from build123d import *

# Parameters (mm, degrees)
SKETCH_1_R      = 1.25
EXTRUDE_1_DEPTH = 3
FILLET_2_R      = 2.5


with BuildPart() as part:
    # Эскиз1 → Бобышка-Вытянуть1 (new body)
    with BuildSketch(Plane.XY):
        with BuildLine():
            Line((-12, -2), (-4.85412196, -2))
            ThreePointArc((-4.85412196, -2), (0, 5.25), (4.85412196, -2))
            Line((4.85412196, -2), (8.261355821, -2))
            ThreePointArc((8.261355821, -2), (2, 8.261355821), (-8.261355821, 2))
            Line((-8.261355821, 2), (-12, 2))
            ThreePointArc((-12, 2), (-14, 0), (-12, -2))
        make_face()
        with Locations((-12, 0)):
            Circle(SKETCH_1_R, mode=Mode.SUBTRACT)
    extrude(amount=EXTRUDE_1_DEPTH)

    # Скругление2
    # the kernel refuses this fillet: 2.5 mm, written as the material it adds along each edge
    with BuildSketch(Plane(origin=(-8.261355821, 2, 0), x_dir=(0.3235599082125896, 0.9462076863973683, 0), z_dir=(0, 0, 1))) as fillet_2_piece_1:
        with BuildLine():
            CenterArc((1.790852834, 2.489434763), FILLET_2_R, 198.878350274, 65.852260083)
            Line((-0.574666382, 1.680534992), (0, 0))
            ThreePointArc((0, 0), (0.780628158, 0.035921806), (1.561256317, 0))
        make_face()
    extrude(amount=3)
    # the kernel refuses this fillet: 2.5 mm, written as the material it takes off along each edge
    with BuildSketch(Plane(origin=(8.261355821, -2, -6.790979044), x_dir=(-1, 0, 0), z_dir=(0, 0, 1))) as fillet_2_2_piece_1:
        with BuildLine():
            CenterArc((2.282225449, -2.5), FILLET_2_R, 90, 94.780191847)
            ThreePointArc((-0.209078872, -2.708333333), (-0.21342859, -1.345760603), (0, 0))
            Line((0, 0), (2.282225449, 0))
        make_face()
    extrude(amount=16.581958087, mode=Mode.SUBTRACT)
    with BuildSketch(Plane(origin=(4.85412196, -2, -7.199330473), x_dir=(0.16240998892159433, 0.9867233632069768, 0), z_dir=(0, 0, 1))) as fillet_2_2_piece_2:
        with BuildLine():
            CenterArc((2.934505681, -2.435474059), FILLET_2_R, 103.045879434, 86.300928937)
            Line((0.467697273, -2.841499031), (0, 0))
            ThreePointArc((0, 0), (1.185088833, -0.135504477), (2.370177665, 0))
        make_face()
    extrude(amount=17.398660947, mode=Mode.SUBTRACT)
    with BuildSketch(Plane(origin=(-4.85412196, -2, -7.199330473), x_dir=(-1, 0, 0), z_dir=(0, 0, 1))) as fillet_2_2_piece_3:
        with BuildLine():
            CenterArc((2.879732189, -2.5), FILLET_2_R, 90, 86.300928937)
            ThreePointArc((0.384940528, -2.338709677), (0.326175697, -1.147347558), (0, 0))
            Line((0, 0), (2.879732189, 0))
        make_face()
    extrude(amount=17.398660947, mode=Mode.SUBTRACT)


solid = part.part
Read the model definition and answer for the solid it produces. Units are mm, in the model's axes. A direction names the side the tool comes from. Give positions to 0.01 mm unless a question says otherwise; leave off trailing zeros. Write each loop counter-clockwise with the first axis right and the second up, starting at its lowest first coordinate (ties: lowest second). Pieces come first, ordered by that corner, then holes. Notation, with made-up numbers: (39.25, 80.25) - (56.25, 80.25) arc R14 ccw to (56.25, 97.25) - close; hole circle Ø11 at (37.25, 45.25). An arc over 180 degrees is marked (long way). Answer in a Markdown table with one row per item. Add a question column.
Item 1: Section D-D, the plane x = 0 is taken. Write down the section's boundary in (y, z), and give its area (3 significant figures).
Item 2: Determine the mould class of faces 4 (the face through (-13.25, 0.05, 1.48)), 5 (the face through (-6, -1.3, 1.5)), 6 (the face through (-3, 5, 3)) for opening direction Y: pulls with the +Y half, pulls with the -Y half, needs draft (parallel to the pull), parting line crosses it, or undercut.
Item 3: Section A-A, the plane z = 1.6 is taken. Write down the section's boundary in (x, y), and give its area (3 significant figures).
Item 4: Flat-ended cylindrical pins translate along their axes: P1, Ø1, axis at y = 5, z = 0.5, coming from the -X side; P2, Ø1, axis at x = -10.5, z = 1.5, coming from the +Y side; P3, Ø1, axis at x = -4.5, z = 1, coming from the +Y side. Find the tip coordinate at first contact, or state that the pin passes through.
Item 5: Find the intervals of material crossed by L1, parallel to X at y = 0.5, z = 1.6; L2, parallel to Y at x = -12, z = 0.95; L3, parallel to X at y = -1, z = 1.2, in increasing order.
Item 6: A tool of negligible diameter and unlimited length cuts with its end or side. For faces 1 (the face through (5.71, -0.97, 1.48)), 2 (the face through (-11, 2, 1)), 3 (the face through (-10, -2, 1)), from which of +Z, -Z, +X, -X, +Y, -Y can it reach the whole face along a straight path? Write none if from no direction.
Item 7: Section C-C, the plane y = 0 is taken. Write down the section's boundary in (x, z), and give its area (3 significant figures).
Item 8: Section B-B, the plane y = 3.25 is taken. Write down the section's boundary in (x, z).
Recorded:
| question | item | result |
|---|---|---|
| 1 | outline | (5.25, 0) - (8.5, 0) - (8.5, 3) - (5.25, 3) - close |
| 1 | area | 9.75 mm2 |
| 2 | face 4 | undercut |
| 2 | face 5 | pulls with the -Y half |
| 2 | face 6 | needs draft |
| 3 | outline | (-12, -2) - (-7.73, -2) arc R2.5 ccw to (-5.24, 0.34) arc R5.25 cw to (5.24, 0.34) arc R2.5 ccw to (6.86, -1.84) arc R2.5 ccw to (8.47, 0.71) arc R8.5 ccw to (-7.76, 3.48) arc R2.5 cw to (-10.04, 2) - (-12, 2) arc R2 ccw to start; hole circle Ø2.5 at (-12, 0) |
| 3 | area | 95.4 mm2 |
| 4 | P1 | stops at x = -7.21 |
| 4 | P2 | stops at y = 2 |
| 4 | P3 | stops at y = 7.5 |
| 5 | L1 | x = -13.94 to -13.15, -10.85 to -5.23, 5.23 to 8.48 |
| 5 | L2 | y = -2 to -1.25, 1.25 to 2 |
| 5 | L3 | x = -13.73 to -12.75, -11.25 to -5.73, 5.73 to 7.98 |
| 6 | face 1 | +Z, -Z, -Y |
| 6 | face 2 | +Z, -Z, -X, +Y |
| 6 | face 3 | +Z, -Z, +X, -X, -Y |
| 7 | outline | (-14, 0) - (-13.25, 0) - (-13.25, 3) - (-14, 3) - close; (-10.75, 0) - (-5.28, 0) - (-5.28, 3) - (-10.75, 3) - close; (5.28, 0) - (8.43, 0) - (8.43, 3) - (5.28, 3) - close |
| 7 | area | 28.1 mm2 |
| 8 | outline | (-7.87, 0) - (-4.12, 0) - (-4.12, 3) - (-7.87, 3) - close; (4.12, 0) - (7.85, 0) - (7.85, 3) - (4.12, 3) - close |
